```python
from build123d import *

# Parameters (mm, degrees)
SKETCH1_W            = 130
SKETCH1_H            = 91
BOSS_EXTRUDE1_DEPTH  = 2.5
SKETCH3_W            = 130
SKETCH3_H            = 2.5
BOSS_EXTRUDE2_DEPTH  = 3
SKETCH2_W            = 130
SKETCH2_H            = 2.5
BOSS_EXTRUDE3_DEPTH  = 3
SKETCH4_W            = 2.5
SKETCH4_H            = 86
BOSS_EXTRUDE4_DEPTH  = 3
SKETCH5_W            = 2.5
SKETCH5_H            = 86
BOSS_EXTRUDE5_DEPTH  = 3
FILLET2_R            = 5
FILLET3_R            = 5
FILLET4_R            = 5
FILLET5_R            = 5
SKETCH7_W            = 2.5
SKETCH7_H            = 68.5
BOSS_EXTRUDE6_DEPTH  = 3
SKETCH8_W            = 24
SKETCH8_H            = 2.5
BOSS_EXTRUDE7_DEPTH  = 11
SKETCH9_W            = 2.5
SKETCH9_H            = 24
BOSS_EXTRUDE8_DEPTH  = 11
SKETCH10_W           = 2.5
SKETCH10_H           = 24
BOSS_EXTRUDE9_DEPTH  = 11
SKETCH11_R           = 3
BOSS_EXTRUDE10_DEPTH = 3
SKETCH12_R           = 1.4
BOSS_EXTRUDE11_DEPTH = 15
SKETCH13_W           = 13
SKETCH13_H           = 23.1
CUT_EXTRUDE1_DEPTH   = 160.702849067
FILLET17_R           = 2
FILLET18_R           = 2
FILLET19_R           = 2
FILLET20_R           = 2
FILLET23_R           = 1
FILLET24_R           = 3
FILLET25_R           = 3
FILLET26_R           = 3


# Some blends are built 0.0001 mm under size
with BuildPart() as part:
    # Sketch1 → Boss-Extrude1 (new body)
    with BuildSketch(Plane.XY):
        with Locations((65, -45.5)):
            Rectangle(SKETCH1_W, SKETCH1_H)
    extrude(amount=BOSS_EXTRUDE1_DEPTH)

    # Sketch3 → Boss-Extrude2 (add)
    with BuildSketch(Plane.XY.offset(2.5)):
        with Locations((65, -89.75)):
            Rectangle(SKETCH3_W, SKETCH3_H)
    extrude(amount=BOSS_EXTRUDE2_DEPTH)

    # Sketch2 → Boss-Extrude3 (add)
    with BuildSketch(Plane.XY.offset(2.5)):
        with Locations((65, -1.25)):
            Rectangle(SKETCH2_W, SKETCH2_H)
    extrude(amount=BOSS_EXTRUDE3_DEPTH)

    # Sketch4 → Boss-Extrude4 (add)
    with BuildSketch(Plane.XY.offset(2.5)):
        with Locations((128.75, -45.5)):
            Rectangle(SKETCH4_W, SKETCH4_H)
    extrude(amount=BOSS_EXTRUDE4_DEPTH)

    # Sketch5 → Boss-Extrude5 (add)
    with BuildSketch(Plane.XY.offset(2.5)):
        with Locations((1.25, -45.5)):
            Rectangle(SKETCH5_W, SKETCH5_H)
    extrude(amount=BOSS_EXTRUDE5_DEPTH)

    # Fillet2
    fillet2_edges = [part.edges().sort_by_distance(p)[0] for p in [
        (130, -91, 2.75),
    ]]
    fillet(fillet2_edges, radius=FILLET2_R)

    # Fillet3
    fillet3_edges = [part.edges().sort_by_distance(p)[0] for p in [
        (130, 0, 2.75),
    ]]
    fillet(fillet3_edges, radius=FILLET3_R)

    # Fillet4
    fillet4_edges = [part.edges().sort_by_distance(p)[0] for p in [
        (0, 0, 2.75),
    ]]
    fillet(fillet4_edges, radius=FILLET4_R)

    # Fillet5
    fillet5_edges = [part.edges().sort_by_distance(p)[0] for p in [
        (0, -91, 2.75),
    ]]
    fillet(fillet5_edges, radius=FILLET5_R)

    # Sketch7 → Boss-Extrude6 (add)
    with BuildSketch(Plane.XY.offset(5.5)):
        with Locations((1.25, -46.75)):
            Rectangle(SKETCH7_W, SKETCH7_H)
    extrude(amount=BOSS_EXTRUDE6_DEPTH)

    # Sketch8 → Boss-Extrude7 (add)
    with BuildSketch(Plane.XY.offset(2.5)):
        with Locations((106.5, -87.25)):
            Rectangle(SKETCH8_W, SKETCH8_H)
    extrude(amount=BOSS_EXTRUDE7_DEPTH)

    # Sketch9 → Boss-Extrude8 (add)
    with BuildSketch(Plane.XY.offset(2.5)):
        with Locations((126.25, -20)):
            Rectangle(SKETCH9_W, SKETCH9_H)
    extrude(amount=BOSS_EXTRUDE8_DEPTH)

    # Sketch10 → Boss-Extrude9 (add)
    with BuildSketch(Plane.XY.offset(2.5)):
        with Locations((3.75, -24)):
            Rectangle(SKETCH10_W, SKETCH10_H)
    extrude(amount=BOSS_EXTRUDE9_DEPTH)

    # Sketch11 → Boss-Extrude10 (add)
    with BuildSketch(Plane.XY.offset(2.5)):
        with Locations(Location((102.5, -20.5, 0), (0, 0, 180))):
            Circle(SKETCH11_R)
    extrude(amount=BOSS_EXTRUDE10_DEPTH)

    # Sketch12 → Boss-Extrude11 (add)
    with BuildSketch(Plane.XY.offset(5.5)):
        with Locations((102.5, -20.5)):
            Circle(SKETCH12_R)
    extrude(amount=BOSS_EXTRUDE11_DEPTH)

    # Sketch13 → Cut-Extrude1 (cut, through all)
    with BuildSketch(Plane.XY.offset(2.5)):
        with Locations((104.5, -62.45)):
            Rectangle(SKETCH13_W, SKETCH13_H)
    extrude(amount=-CUT_EXTRUDE1_DEPTH, mode=Mode.SUBTRACT)

    # Fillet17
    fillet17_edges = [part.edges().sort_by_distance(p)[0] for p in [
        (98, -74, 1.25),
    ]]
    fillet(fillet17_edges, radius=FILLET17_R)

    # Fillet18
    fillet18_edges = [part.edges().sort_by_distance(p)[0] for p in [
        (98, -50.9, 1.25),
    ]]
    fillet(fillet18_edges, radius=FILLET18_R)

    # Fillet19
    fillet19_edges = [part.edges().sort_by_distance(p)[0] for p in [
        (111, -50.9, 1.25),
    ]]
    fillet(fillet19_edges, radius=FILLET19_R)

    # Fillet20
    fillet20_edges = [part.edges().sort_by_distance(p)[0] for p in [
        (111, -74, 1.25),
    ]]
    fillet(fillet20_edges, radius=FILLET20_R)

    # Fillet23
    fillet23_edges = [part.edges().sort_by_distance(p)[0] for p in [
        (104.5, -74, 0),
        (98.585786438, -73.414213562, 0),
        (98, -62.45, 0),
        (98.585786438, -51.485786438, 0),
        (104.5, -50.9, 0),
        (110.414213562, -51.485786438, 0),
        (111, -62.45, 0),
        (110.414213562, -73.414213562, 0),
    ]]
    fillet(fillet23_edges, radius=FILLET23_R)

    # Fillet24
    fillet24_edges = [part.edges().sort_by_distance(p)[0] for p in [
        (128.535533906, -89.535533906, 0),
        (130, -45.5, 0),
        (128.535533906, -1.464466094, 0),
        (0, -45.5, 0),
        (65, 0, 0),
        (1.464466094, -1.464466094, 0),
        (65, -91, 0),
        (1.464466094, -89.535533906, 0),
    ]]
    fillet(fillet24_edges, radius=FILLET24_R)

    # Fillet25
    # the kernel refuses this fillet: 3 mm, written as the material it adds along each edge
    with BuildSketch(Plane(origin=(102.5, -20.5, 5.5), x_dir=(1, 0, 0), z_dir=(0, -1, 0))) as fillet25_piece_1:
        with BuildLine():
            CenterArc((4.4, 2.653299832), FILLET25_R, 180, 62.181860715)
            Line((1.4, 2.653299832), (1.34, 2.653299832))
            Line((1.34, 2.653299832), (1.34, 0))
            Line((1.34, 0), (1.4, -0.06))
            ThreePointArc((1.4, -0.06), (2.2, -0.06), (2.972, -0.053065997))
            Line((2.972, -0.053065997), (3, 0))
        make_face()
    revolve(axis=Axis((102.5, -20.5, 5.5), (0, 0, 1)))

    # Fillet26
    fillet26_edges = [part.edges().sort_by_distance(p)[0] for p in [
        (105.5, -20.5, 2.5),
    ]]
    fillet(fillet26_edges, radius=FILLET26_R - 0.0001)  # a hair under: the kernel refuses the full size


solid = part.part
```
Verification items for the finished model (mm, model axes). A direction names the side the tool comes from. Round coordinates to 2 decimals unless told otherwise and drop trailing zeros. Write each loop counter-clockwise with the first axis right and the second up, starting at its lowest first coordinate (ties: lowest second). Pieces come first, ordered by that corner, then holes.
1. Access from +Z, -Z, +X, -X, +Y, -Y to the whole of each face (thin tool, end or side, straight path). Record for faces 5 (the flat face through (127.5, -5, 4)), 6 (the flat face through (1, -46, 8.5)), 7 (the flat face through (106, -88.5, 9)).
2. Gauge pin test, flat ends, axial feed: P1, Ø8, axis at x = 36.5, y = -17.5, coming from the +Z side; P2, Ø1.2, axis at y = -86.5, z = 9.5, coming from the -X side; P3, Ø12, axis at y = -22, z = 15, coming from the -X side. Record the tip position at first contact, or that the pin passes through.
3. Scan lines: L1, parallel to Y at x = 114.5, z = 5.25; L2, parallel to X at y = -18, z = 5.25; L3, parallel to Z at x = 114.5, y = -52. Record each from-to range of solid material in increasing order.
4. Section check A-A on y = -59. Enter the section's corners in (x, z), plus the area to 3 significant figures.
5. Section check D-D on x = 26. Enter the section's corners in (y, z), plus the area to 3 significant figures.
6. Section check C-C on y = -84.5. Enter the section's corners in (x, z).
7. Draft check along X on faces 1 (the flat face through (48, -88.5, 4)), 2 (the flat face through (1, -12.5, 7)), 3 (the flat face through (0, -46, 6)), 4 (the flat face through (130, -46, 4)). Enter one of: +X half, -X half, draft (parallel to the pull), parting line (faces both ways), or undercut.
Answer:
1. face 5: +Z
1. face 6: +Z, -X, +Y, -Y
1. face 7: +Z, +X, -X, -Y
2. P1: stops at z = 2.5
2. P2: stops at x = 94.5
2. P3: stops at x = 2.5
3. L1: y = -91 to -86, -2.5 to 0
3. L2: x = 0 to 5, 100.82 to 104.18, 125 to 130
3. L3: z = 0 to 2.5
4. outline: (0, 3) arc R3 ccw to (3, 0) - (97, 0) arc R1 ccw to (98, 1) - (98, 2.5) - (2.5, 2.5) - (2.5, 8.5) - (0, 8.5) - close; (111, 1) arc R1 ccw to (112, 0) - (127, 0) arc R3 ccw to (130, 3) - (130, 5.5) - (127.5, 5.5) - (127.5, 2.5) - (111, 2.5) - close
4. area: 311 mm2
5. outline: (-91, 3) arc R3 ccw to (-88, 0) - (-3, 0) arc R3 ccw to (0, 3) - (0, 5.5) - (-2.5, 5.5) - (-2.5, 2.5) - (-88.5, 2.5) - (-88.5, 5.5) - (-91, 5.5) - close
5. area: 239 mm2
6. outline: (0, 3) arc R3 ccw to (3, 0) - (127, 0) arc R3 ccw to (130, 3) - (130, 5.5) - (127.5, 5.5) - (127.5, 2.5) - (2.5, 2.5) - (2.5, 5.5) - (0, 5.5) - close
7. face 1: undercut
7. face 2: draft
7. face 3: -X half
7. face 4: +X half
